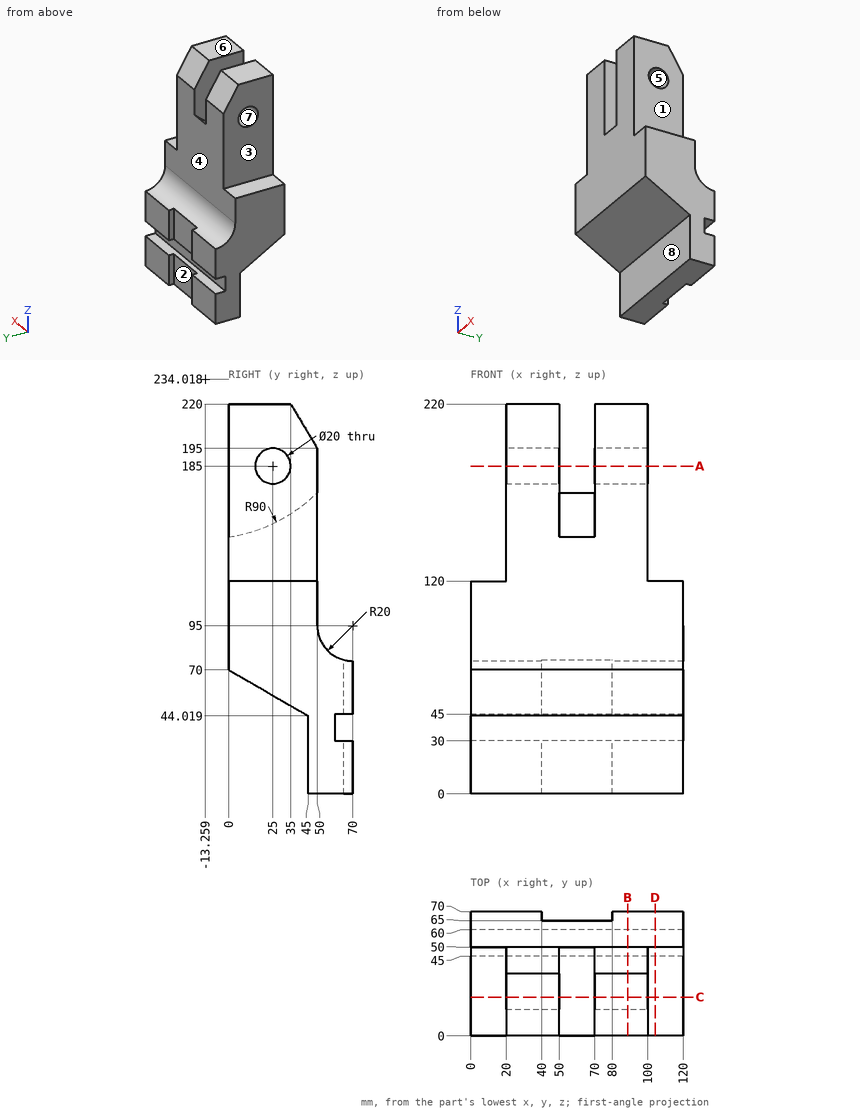
Geometry check sheet. Reference: drawing and pictorial views, mm from the part's lowest x, y, z. A direction names the side the tool comes from. Give positions to 0.01 mm unless a question says otherwise; leave off trailing zeros. Order: outer loops, then holes, each group sorted by start corner. A loop starts at its lowest first (then second) coordinate and runs counter-clockwise, first axis right, second up. Notation, with made-up numbers: M 67.5,0.5 L 118.5,0.5 A34 ccw 118.5,34.5 Z; hole C 8,67.5 d9. An arc over 180 degrees is marked long. Answer as a JSON object with one key per item and string values. Group by question number.
1) Cross-section at C-C (y = 22). Enter the section's corners in (x, z).
2) Cross-section at A-A (z = 185). Enter the section's corners in (x, y), then the cut area to 3 significant figures.
3) Access from +Z, -Z, +X, -X, +Y, -Y to the whole of each face (thin tool, end or side, straight path). Record for the marked faces 1, 2, 3, 4 and 5.
4) Cross-section at D-D (x = 104). Enter the section's corners in (y, z).
5) Scan lines: line 1 along X through (y, z) = (46, 182.5); line 2 along Z through (x, y) = (90, 25); line 3 along Y through (x, z) = (20.5, 146). Record each from-to range of solid material in increasing order. Write a range as [from, to].
6) Cross-section at B-B (x = 88.5). Enter the section's corners in (y, z), then the cut area to 3 significant figures.
7) Mould release check, pull along Z, two halves, no side actions. Record for the marked faces 6, 7 and 8: released by +Z, released by -Z, zero draft, split by the parting line, or undercut.
8) Depth check by flat-ended pin: pin 1 Ø2 at (x, z) = (72, 35) entering from -Y; pin 2 Ø24 at (x, z) = (53.5, 12.5) entering from +Y; pin 3 Ø3 at (x, z) = (81.5, 175) entering from +Y; pin 4 Ø16 at (y, z) = (25, 185) entering from +X. Enter the tip coordinate at first touch or a pass-through.
Result sheet:
{
 "1": {"outline": "M 0,57.3 L 120,57.3 L 120,120 L 100,120 L 100,175.46 L 70,175.46 L 70,151.21 L 50,151.21 L 50,175.46 L 20,175.46 L 20,120 L 0,120 Z; M 20,194.54 L 50,194.54 L 50,220 L 20,220 Z; M 70,194.54 L 100,194.54 L 100,220 L 70,220 Z"},
 "2": {"outline": "M 20,0 L 50,0 L 50,15 L 20,15 Z; M 20,35 L 50,35 L 50,50 L 20,50 Z; M 70,0 L 100,0 L 100,15 L 70,15 Z; M 70,35 L 100,35 L 100,50 L 70,50 Z", "area": "1,800 mm2"},
 "3": {"face 1": "+Z, +X, +Y, -Y", "face 2": "+Z, -Z, +Y", "face 3": "+Z, -X, +Y, -Y", "face 4": "+Z, +X, -X, +Y", "face 5": "+X, -X"},
 "4": {"outline": "M 0,70 L 45,44.02 L 45,0 L 70,0 L 70,30 L 60,30 L 60,45 L 70,45 L 70,75 A20 cw 50,95 L 50,120 L 0,120 Z"},
 "5": {"line 1": "x = [20, 50], [70, 100]", "line 2": "z = [55.57, 175], [195, 220]", "line 3": "y = [0, 50]"},
 "6": {"outline": "M 0,70 L 45,44.02 L 45,0 L 70,0 L 70,30 L 60,30 L 60,45 L 70,45 L 70,75 A20 cw 50,95 L 50,195 L 35,220 L 0,220 Z; hole C 25,185 d20", "area": "9,370 mm2"},
 "7": {"face 6": "released by +Z", "face 7": "undercut", "face 8": "zero draft"},
 "8": {"pin 1": "stops at y = 45", "pin 2": "stops at y = 65", "pin 3": "stops at y = 50", "pin 4": "passes through"}
}
